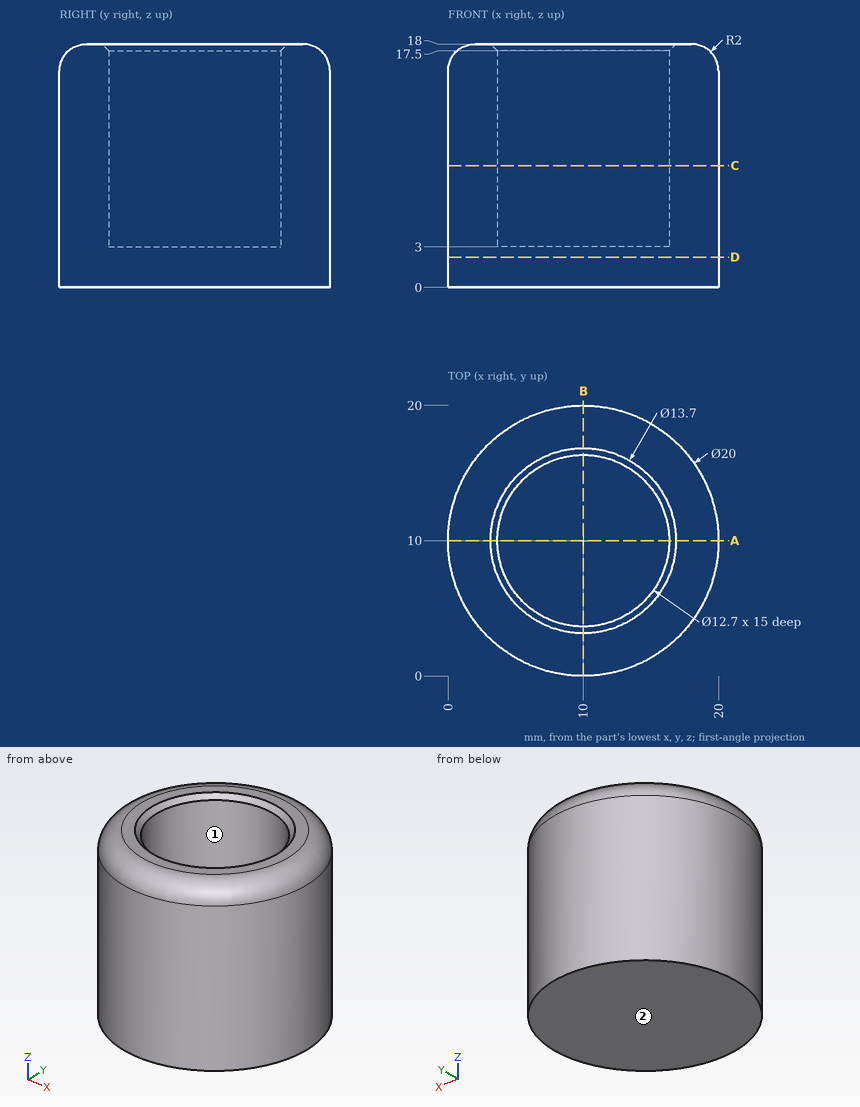
Verification items for this drawing (mm, ordinates from the low corner). A direction names the side the tool comes from. Give positions to 0.01 mm unless a question says otherwise; leave off trailing zeros. Loops run counter-clockwise (first coordinate to the right, second up) from the corner with the lowest first, then second, coordinate; pieces in that order, holes last. Notation, with made-up numbers: M 56.25,39.5 L 106.25,39.5 A22 ccw 106.25,70.5 Z; hole C -28,8.25 d7. An arc over 180 degrees is marked long. Write item = value, one per line. Start each with the question number.
1. Go/stop test with flat-tipped pins: P1, Ø4, axis at x = 11, y = 11, coming from the +Z side; P2, Ø5, axis at x = 11, z = 8, coming from the +Y side; P3, Ø1, axis at y = 9, z = 14, coming from the +X side; P4, Ø1, axis at y = 6.5, z = 3.5, coming from the -X side. Record where each tip stops, or that it passes through.
2. Thickness scan on probe 1 along X at (y, z) = (10, 8.5); probe 2 along Y at (x, z) = (8.5, 13.5). Record the ranges inside material, lowest first.
3. Section check C-C, the plane z = 9. Enter the section's corners in (x, y), plus the area to 3 significant figures.
4. Section check D-D, the plane z = 2.25. Enter the section's corners in (x, y), plus the area to 3 significant figures.
5. Section check A-A, the plane y = 10. Enter the section's corners in (x, z).
6. Tool access check on the marked faces 1 and 2. Record the directions out of +Z, -Z, +X, -X, +Y, -Y that give a thin tool (end or side, any length) a straight path to the whole face; none if there is none.
Values follow:
q1.P1 = 3
q1.P2 = 20
q1.P3 = 19.99
q1.P4 = 0.46
q2.probe_1 = 0 to 3.65, 16.35 to 20
q2.probe_2 = 0.11 to 3.83, 16.17 to 19.89
q3.outline = C 10,10 d20; hole C 10,10 d12.7
q3.area = 187 mm^2
q4.outline = C 10,10 d20
q4.area = 314 mm^2
q5.outline = M 0,0 L 20,0 L 20,16 A2 ccw 18,18 L 16.85,18 L 16.35,17.5 L 16.35,3 L 3.65,3 L 3.65,17.5 L 3.15,18 L 2,18 A2 ccw 0,16 Z
q6.face_1 = +Z
q6.face_2 = -Z, +X, -X, +Y, -Y
